Design review of the part built by this model. Coordinates are the model's own, in mm. A direction names the side the tool comes from. Coordinates: 2 decimals unless noted, no trailing zeros. Order: outer loops, then holes, each group sorted by start corner. A loop starts at its lowest first (then second) coordinate and runs counter-clockwise, first axis right, second up. Notation, with made-up numbers: M 80.5,84 L 122.5,84 A16 cw 122.5,105 Z; hole C 58.5,-33.5 d8. An arc over 180 degrees is marked long. Answer in a Markdown table with one row per item.
from build123d import *

# Parameters (mm, degrees)
FILLET_1_R          = 0.3
CUT_EXTRUDE_1_DEPTH = 2.4
CHAMFER_1_SIZE      = 0.2


with BuildPart() as part:
    # 草图1 → 旋转1 (revolve)
    with BuildSketch(Plane(origin=(0, 0, 0), x_dir=(0, 0, -1), z_dir=(1, 0, 0))):
        Polygon((0, 0), (0, 2), (-8, 2), (-8, 2.5), (-38, 2.5), (-38, 4.5), (-41.5, 4.5), (-41.5, 0), align=None)
    revolve(axis=Axis((0, 0, 0), (0, 0, 1)))

    # 圆角1
    fillet_1_edges = [part.edges().sort_by_distance(p)[0] for p in [
        (0, -4.5, 41.5),
        (0, -4.5, 38),
    ]]
    fillet(fillet_1_edges, radius=FILLET_1_R)

    # 草图2 → 切除-拉伸1 (cut)
    with BuildSketch(Plane.XY.offset(41.5)):
        Polygon((1.732050808, 0), (0.866025404, 1.5), (-0.866025404, 1.5), (-1.732050808, 0), (-0.866025404, -1.5), (0.866025404, -1.5), align=None)
    extrude(amount=-CUT_EXTRUDE_1_DEPTH, mode=Mode.SUBTRACT)

    # 倒角1
    chamfer_1_edges = [part.edges().sort_by_distance(p)[0] for p in [
        (0, -2.5, 8),
    ]]
    chamfer(chamfer_1_edges, length=CHAMFER_1_SIZE)


solid = part.part
(1) Draft analysis for pull direction X (two halves, no side actions). For faces 1 (the flat face through (0, 0, 0)), 2 (the flat face through (0, -1.5, 40)), 3 (the flat face through (-1.305, -0.74, 40.317)), 4 (the cylindrical face through (-4.46, -0.59, 39.77)), state which applies: pulls with the +X half, pulls with the -X half, needs draft (parallel to the pull), parting line crosses it, or undercut.
Return value:
| item | result |
|---|---|
| face 1 | needs draft |
| face 2 | undercut |
| face 3 | undercut |
| face 4 | parting line crosses it |
(2) Add section C-C, the plane z = 36. Give the boundary of the cut face in (x, y), and give its area (3 significant figures).
Return value:
| item | result |
|---|---|
| outline | C 0,0 d5 |
| area | 19.6 mm2 |
(3) Add section A-A, the plane x = 0. Give the boundary of the cut face in (y, z), and give its area (3 significant figures).
Return value:
| item | result |
|---|---|
| outline | M -4.5,38.3 A0.3 ccw -4.2,38 L -2.5,38 L -2.5,8.2 L -2.3,8 L -2,8 L -2,0 L 2,0 L 2,8 L 2.3,8 L 2.5,8.2 L 2.5,38 L 4.2,38 A0.3 ccw 4.5,38.3 L 4.5,41.2 A0.3 ccw 4.2,41.5 L 1.5,41.5 L 1.5,39.1 L -1.5,39.1 L -1.5,41.5 L -4.2,41.5 A0.3 ccw -4.5,41.2 Z |
| area | 206 mm2 |
(4) For faces 5 (the flat face through (0, 0, 39.1)), 6 (the flat face through (0, 2, 41.5)), 7 (the cylindrical face through (2, 0, 4)), list the 3-axis set-ups (+Z, -Z, +X, -X, +Y, -Y) from which the entire face can be reached by the end or side of a thin tool; tool diameter is ignored.
Return value:
| item | result |
|---|---|
| face 5 | +Z |
| face 6 | +Z, +X, -X, +Y, -Y |
| face 7 | -Z |
(5) Add section B-B, the plane z = 7.5. Give the boundary of the cut face in (x, y), and give its area (3 significant figures).
Return value:
| item | result |
|---|---|
| outline | C 0,0 d4 |
| area | 12.6 mm2 |
(6) For line 1 along Y through (x, z) = (1.5, 34); line 2 along Z through (x, y) = (3, -0.5), list the stretches that pass through material, from the lowest coordinate up. Write a range as from..to.
Return value:
| item | result |
|---|---|
| line 1 | y = -2..2 |
| line 2 | z = 38..41.5 |
(7) Insertion check: pin 1 Ø1 at (x, y) = (2.5, 0.5) entering from -Z; pin 2 Ø4 at (x, z) = (3, 12) entering from -Y; pin 3 Ø5 at (y, z) = (-0.5, 30.5) entering from +X. Each pin has a flat end and moves straight along its axis. Give the tip position at first contact, or say it passes through.
Return value:
| item | result |
|---|---|
| pin 1 | stops at z = 8 |
| pin 2 | stops at y = -2.29 |
| pin 3 | stops at x = 2.5 |
